```python
from build123d import *

# Parameters (mm, degrees)
F0_R     = 27.94
F0_R_2   = 2.286
F1_DEPTH = 2.794
F4_R     = 3.81
F5_DEPTH = 12.7


# Not quite as in the source:
# - a feature names something its author has since deleted; it is built from what else it names


with BuildPart() as f1:
    # F0 (on Top) → F1 (new body, symmetric)
    with BuildSketch(Plane.XY):
        Circle(F0_R)
        with BuildLine():
            ThreePointArc((7.4038372238, 22.9660639719), (19.5052748277, 14.2056732996), (24.13, 0))
            ThreePointArc((24.13, 0), (23.8372400211, -3.7473841781), (22.9660639719, -7.4038372238))
            ThreePointArc((22.9660639719, -7.4038372238), (14.2056732996, -19.5052748277), (0, -24.13))
            ThreePointArc((0, -24.13), (-3.7473841781, -23.8372400211), (-7.4038372238, -22.9660639719))
            ThreePointArc((-7.4038372238, -22.9660639719), (-19.5052748277, -14.2056732996), (-24.13, 0))
            ThreePointArc((-24.13, 0), (-23.8372400211, 3.7473841781), (-22.9660639719, 7.4038372238))
            ThreePointArc((-22.9660639719, 7.4038372238), (-14.2056732996, 19.5052748277), (0, 24.13))
            ThreePointArc((0, 24.13), (3.7473841781, 23.8372400211), (7.4038372238, 22.9660639719))
        make_face(mode=Mode.SUBTRACT)
        with BuildLine():
            ThreePointArc((22.9660639719, -7.4038372238), (23.8372400211, -3.7473841781), (24.13, 0))
            ThreePointArc((24.13, 0), (13.395886303, 8.0244732927), (0, 7.62))
            ThreePointArc((0, 7.62), (2.0157431704, 16.1065414645), (7.4038372238, 22.9660639719))
            ThreePointArc((7.4038372238, 22.9660639719), (3.7473841781, 23.8372400211), (0, 24.13))
            ThreePointArc((0, 24.13), (-8.0244732927, 13.395886303), (-7.62, 0))
            ThreePointArc((-7.62, 0), (-16.1065414645, 2.0157431704), (-22.9660639719, 7.4038372238))
            ThreePointArc((-22.9660639719, 7.4038372238), (-23.8372400211, 3.7473841781), (-24.13, 0))
            ThreePointArc((-24.13, 0), (-13.395886303, -8.0244732927), (0, -7.62))
            ThreePointArc((0, -7.62), (-2.0157431704, -16.1065414645), (-7.4038372238, -22.9660639719))
            ThreePointArc((-7.4038372238, -22.9660639719), (-3.7473841781, -23.8372400211), (0, -24.13))
            ThreePointArc((0, -24.13), (8.0244732927, -13.395886303), (7.62, 0))
            ThreePointArc((7.62, 0), (16.1065414645, -2.0157431704), (22.9660639719, -7.4038372238))
        make_face()
        Polygon((3.1270369256, 6.3063403068), (7.0249693735, 0.4450767373), (3.8979324478, -5.8612635696), (-3.1270369256, -6.3063403068), (-7.0249693735, -0.4450767373), (-3.8979324478, 5.8612635696), align=None, mode=Mode.SUBTRACT)
        Polygon((3.8979324478, -5.8612635696), (7.0249693735, 0.4450767373), (3.1270369256, 6.3063403068), (-3.8979324478, 5.8612635696), (-7.0249693735, -0.4450767373), (-3.1270369256, -6.3063403068), align=None)
        Circle(F0_R_2, mode=Mode.SUBTRACT)
    extrude(amount=F1_DEPTH, both=True)

    # F2 (on Front) → F3 (revolve, cut)
    with BuildSketch(Plane.XZ):
        with BuildLine():
            Line((27.94, -1.5875), (27.94, 0))
            Line((27.94, 0), (26.3525, 0))
            ThreePointArc((26.3525, 0), (26.8174679849, -1.1225320151), (27.94, -1.5875))
        make_face()
        with BuildLine():
            Line((26.3525, 0), (27.94, 0))
            Line((27.94, 0), (27.94, 1.5875))
            ThreePointArc((27.94, 1.5875), (26.8174679849, 1.1225320151), (26.3525, 0))
        make_face()
    revolve(axis=Axis((0, 0, -0.2561928704), (0, 0, -1)), mode=Mode.SUBTRACT)

    # F4
    f4_edges = [f1.edges().sort_by_distance(p)[0] for p in [
        (-7.62, 0, 0),
        (0, 7.62, 0),
        (7.62, 0, 0),
        (0, -7.62, 0),
    ]]
    fillet(f4_edges, radius=F4_R)

    # F0 (on Top) → F5 (cut)
    with BuildSketch(Plane.XY):
        Polygon((3.8979324478, -5.8612635696), (7.0249693735, 0.4450767373), (3.1270369256, 6.3063403068), (-3.8979324478, 5.8612635696), (-7.0249693735, -0.4450767373), (-3.1270369256, -6.3063403068), align=None)
        Circle(F0_R_2, mode=Mode.SUBTRACT)
    extrude(amount=-F5_DEPTH, mode=Mode.SUBTRACT)


solid = f1.part
```
For this review, take the finished solid that the model builds, in its own axes (mm). A direction names the side the tool comes from. Round coordinates to 2 decimals unless told otherwise and drop trailing zeros. One line per question, with ' | ' between items. Start each with the question number.
1) Mouldability with a two-part tool opening along X and no side actions: class faces 1 (the cylindrical face through (-3.64, 27.7, 2.2)), 2 (the cylindrical face through (14.377, -19.379, 0.039)), 3 (the flat face through (6, 0, 2.794)) as +X half, -X half, draft (parallel to the pull), parting line (faces both ways), or undercut.
2) Machinability: for faces 4 (the flat face through (5.44, -2.75, -1.38)), 5 (the cylindrical face through (-3.577, -18.795, 0.039)), 6 (the flat face through (6, -6, -2.794)), which of the approach directions +Z, -Z, +X, -X, +Y, -Y give a long, thin tool a straight path to every point of the face, cutting with its end or side? Answer none if there is none.
3) Add section A-A (x = -19.5). Count the separate pieces of the cut face and the enclosed holes in it, and give its area (3 significant figures).
4) Wall thickness on line 1 along Y through (x, z) = (-17, -1.9); line 2 along Y through (x, z) = (17, -1.05); line 3 along X through (y, z) = (-3.5, -1.35): over which ranges is each line inside the solid? List them lowest first.
5) For pin 1 Ø12 at (x, y) = (12, -1) entering from -Z; pin 2 Ø1 at (x, z) = (-1.5, 1.5) entering from +Y; pin 3 Ø1 at (y, z) = (-10.5, -2) entering from -X; pin 4 Ø3 at (x, z) = (-6.5, 1) entering from +Y, all flat-tipped, find the tip position at first contact; note any pin that passes through.
Reported:
1) face 1: parting line | face 2: undercut | face 3: draft
2) face 4: -Z | face 5: +Z, -Z | face 6: -Z, +X, -X, +Y, -Y
3) separate pieces: 3 | enclosed holes: 0 | area: 104 mm²
4) line 1: y = -22.17 to -17.12, -6.49 to 2.47, 17.12 to 22.17 | line 2: y = -20.65 to -17.12, -2.47 to 6.49, 17.12 to 20.65 | line 3: x = -26.88 to -23.87, -21.14 to -4.99, 5.07 to 9.02, 18.68 to 26.88
5) pin 1: stops at z = -2.79 | pin 2: stops at y = 27.92 | pin 3: stops at x = -26.09 | pin 4: stops at y = 27.47
